Autodesk Inventor part; units mm, degrees
ref_plane "YZ Plane" through (0, 0, 0) normal (1, 0, 0) x (0, 1, 0)
ref_plane "XZ Plane" through (0, 0, 0) normal (0, 1, 0) x (-1, 0, 0)
ref_plane "XY Plane" through (0, 0, 0) normal (0, 0, 1) x (1, 0, 0)
sketch "スケッチ1" plane through (0, 0, 0) normal (1, 0, 0) x (0, 1, 0)
  circle A0 centre (0, 0) radius 5
  circle A1 centre (0, 0) radius 13
  dimension "d0" = 10
  dimension "d1" = 26
extrude "押し出し1" add sketch "スケッチ1" along normal blind 8
sketch "スケッチ2" plane through (8, 0, 0) normal (1, 0, 0) x (0, 0, -1)
  circle A0 centre (0, 0) radius 6
  circle A1 centre (0, 0) radius 12
  dimension "d4" = 12
  dimension "d5" = 24
extrude "押し出し2" cut sketch "スケッチ2" against normal blind 0.1
sketch "スケッチ3" plane through (0, 0, 0) normal (-1, 0, 0) x (0, 0, 1)
  circle A0 centre (0, 0) radius 6
  circle A1 centre (0, 0) radius 12
  dimension "d8" = 12
  dimension "d9" = 24
extrude "押し出し3" cut sketch "スケッチ3" against normal blind 0.1
properties part number "Bearing_6000ZZ" material "鋼、炭素鋼"
Here's how the part is built. I have some questions about the finished solid (model axes, mm). A direction names the side the tool comes from. Coordinates: 2 decimals unless noted, no trailing zeros. Write each loop counter-clockwise with the first axis right and the second up, starting at its lowest first coordinate (ties: lowest second). Pieces come first, ordered by that corner, then holes. Notation, with made-up numbers: (-10.5, 38.5) - (27.5, 38.5) arc R35 ccw to (27.5, 75.5) - close; hole circle Ø7 at (-5.75, -9.5). An arc over 180 degrees is marked (long way). One line per item, written item: value.
1) Suppose I cut it at A-A on z = 0. Write out the boundary of the cut face in (x, y), and give its area (3 significant figures).
Model answer:
outline: (0, -13) - (8, -13) - (8, -12) - (7.9, -12) - (7.9, -6) - (8, -6) - (8, -5) - (0, -5) - (0, -6) - (0.1, -6) - (0.1, -12) - (0, -12) - close; (0, 5) - (8, 5) - (8, 6) - (7.9, 6) - (7.9, 12) - (8, 12) - (8, 13) - (0, 13) - (0, 12) - (0.1, 12) - (0.1, 6) - (0, 6) - close
area: 126 mm²
2) I'm going to push flat-ended pins straight in: P1, Ø1.5, axis at y = 2.5, z = -10.5, coming from the -X side; P2, Ø1, axis at y = -3, z = -3, coming from the -X side; P3, Ø2, axis at x = 6, z = -4.5, coming from the +Y side; P4, Ø1.5, axis at x = 4, y = -10.5, coming from the -Z side. Where does each tip first touch, or does it pass through?
Model answer:
P1: stops at x = 0.1
P2: passes through
P3: stops at y = 12.52
P4: stops at z = -8.6
3) On a 3-axis mill with a long thin cutter (end or side, diameter ignored), from which of +Z, -Z, +X, -X, +Y, -Y can I reach the whole of each face in a straight line? I mean faces 4 (the flat face through (0, -4, 4)), 5 (the flat face through (0.1, -2, -6)). Say none if no direction works.
Model answer:
face 4: +Z, -Z, -X, +Y, -Y
face 5: -X
4) Suppose I cut it at C-C on z = -6.5. Write out the boundary of the cut face in (x, y).
Model answer:
outline: (0, -11.26) - (8, -11.26) - (8, -10.09) - (7.9, -10.09) - (7.9, 10.09) - (8, 10.09) - (8, 11.26) - (0, 11.26) - (0, 10.09) - (0.1, 10.09) - (0.1, -10.09) - (0, -10.09) - close
5) Suppose I cut it at D-D on y = 9. Write out the boundary of the cut face in (x, z).
Model answer:
outline: (0, -9.38) - (8, -9.38) - (8, -7.94) - (7.9, -7.94) - (7.9, 7.94) - (8, 7.94) - (8, 9.38) - (0, 9.38) - (0, 7.94) - (0.1, 7.94) - (0.1, -7.94) - (0, -7.94) - close
6) I need wall thicknesses on line 1 along Z through (x, y) = (3.75, 0); line 2 along X through (y, z) = (7.5, 8); line 3 along Y through (x, z) = (1.25, -0.25). Which ranges of each line are inside material? Lowest first, please.
Model answer:
line 1: z = -13 to -5, 5 to 13
line 2: x = 0.1 to 7.9
line 3: y = -13 to -4.99, 4.99 to 13
7) We'd pull the mould along Y, two halves only. Please class faces 1 (the flat face through (8, -4, 4)), 2 (the cylindrical face through (3.944, -10.316, 7.91)), 3 (the flat face through (7.9, -2, 6)): pulls with the +Y half, pulls with the -Y half, needs draft (parallel to the pull), parting line crosses it, or undercut.
Model answer:
face 1: needs draft
face 2: parting line crosses it
face 3: undercut
